Build history of the part. All positions in model axes, mm. A direction names the side the tool comes from. Give positions to 0.01 mm unless a question says otherwise; leave off trailing zeros. Write each loop counter-clockwise with the first axis right and the second up, starting at its lowest first coordinate (ties: lowest second). Pieces come first, ordered by that corner, then holes.
Autodesk Inventor part; units mm, degrees
ref_plane "YZ Plane" through (0, 0, 0) normal (1, 0, 0) x (0, 1, 0)
ref_plane "XZ Plane" through (0, 0, 0) normal (0, 1, 0) x (-1, 0, 0)
ref_plane "XY Plane" through (0, 0, 0) normal (0, 0, 1) x (1, 0, 0)
sketch "Sketch1" plane through (0, 0, 0) normal (0, 0, 1) x (1, 0, 0)
  line L0 (0, 0) -> (-40, 0)
  line L1 (-40, 0) -> (-40, -132)
  line L2 (-40, -132) -> (0, -132)
  line L3 (0, -132) -> (0, 0)
  line L4 (-30, -105) -> (-10, -105) construction
  line L5 (-10, -105) -> (-10, -125) construction
  line L6 (-10, -125) -> (-30, -125) construction
  line L7 (-30, -125) -> (-30, -105) construction
  line L8 (-20, -105) -> (-20, -80) construction
  line L9 (-20, -80) -> (-20, -60) construction
  line L10 (-20, -60) -> (-20, -40) construction
  line L11 (-20, -40) -> (-20, -20) construction
  line L12 (-20, -20) -> (-20, 0) construction
  dimension "d0" = 20
  dimension "d1" = 20
  dimension "d2" = 25
  dimension "d3" = 20
  dimension "d4" = 7
  dimension "d5" = 10
extrude "Plate1" add sketch "Sketch1" along normal blind 2.286
hole "Hole1" at (-20, -80, 0) at (-20, -60, 0) at (-20, -40, 0) at (-20, -20, 0) at (-10, -125, 0) at (-10, -105, 0) at (-30, -105, 0) at (-30, -125, 0) direction (0, 0, 1) diameter 3.4 end through all
sketch "Sketch2" plane through (-37.714, 0, 2.286) normal (-1, 0, 0) x (0, -1, 0)
  line L0 (132, 0) -> (0, 0)
  line L1 (0, 0) -> (0, -12.7)
  line L2 (0, -12.7) -> (132, -12.7)
  line L3 (132, -12.7) -> (132, 0)
edge flange "Flange1" height 12.7 angle 90 thickness 2.286 bend radius 2.286 thickness toward (-1, 0, 0) relief tear relief width 2.286 relief depth 1.143 corner gap 2.286 corner form 0 edges at (-40, -66, 0) (0, -66, 0) wall of the first edge with corners at (-37.714, -132, 2.286) (-37.714, 0, 2.286) (-37.714, 0, -10.414) (-37.714, -132, -10.414)
bend "Bend1"
corner "Corner1"
equation "\"d12\" = Thickness"
equation "\"d6\" = Thickness"
equation "\"d14\" = BendReliefWidth"
equation "\"d15\" = BendReliefDepth"
equation "\"d16\" = MinimumRemnant"
equation "\"d17\" = TransitionRadius"
equation "\"d20\" = BendRadius"
equation "\"d21\" = CornerReliefSize"
equation "\"d22\" = GapSize"
equation "\"d23\" = JacobiRadiusSize"
equation "\"BendRadius\" = Thickness"
equation "\"BendReliefWidth\" = Thickness"
equation "\"BendReliefDepth\" = 0.5 * Thickness"
equation "\"CornerReliefSize\" = 4 * Thickness"
equation "\"MinimumRemnant\" = 2 * Thickness"
equation "\"TransitionRadius\" = BendRadius"
equation "\"JacobiRadiusSize\" = BendRadius"
equation "\"GapSize\" = Thickness"
properties part number "Bed Mount"
(1) Drop flat-ended pins along their axis: pin 1 (4 mm diameter, centred on x = -22, y = -32, fed in from -Z); pin 2 (3 mm diameter, centred on x = -35.5, y = -40.5, fed in from -Z); pin 3 (6 mm diameter, centred on x = -33, z = -7.5, fed in from +Y). Give the stop position or say it passes through.
(2) Saw through at B-B, the plane z = -4. List the corners of the cut face in (x, y), plus the area to 3 significant figures.
(3) Saw through at C-C, the plane y = -20. List the corners of the cut face in (x, z), plus the area to 3 significant figures.
(4) Saw through at A-A, the plane x = -10. List the corners of the cut face in (y, z), plus the area to 3 significant figures.
(5) Probe line 1 (Y direction, x = -30, z = 0.55); line 2 (X direction, y = -23, z = -9.5); line 3 (X direction, y = -105, z = 1.1). List the from-to ranges inside material, lowest first.
(6) Saw through at D-D, the plane y = -105. List the corners of the cut face in (x, z).
(7) 3-axis set-ups, long thin cutter, end or side, ignore diameter. For faces 5 (the face through (-20, -65, 0)), 6 (the face through (-22, 0, 1)): which of +Z, -Z, +X, -X, +Y, -Y reach the whole face in a straight line?
(8) Mould opens along X. For faces 1 (the face through (-39, -65, -10.414)), 2 (the face through (-30.07, -106.7, 1.16)), 3 (the face through (-38.7, -65.08, 0.91)), 4 (the face through (0, -67, -6)) say: +X half, -X half, draft (parallel to the pull), parting line (faces both ways), or undercut.
Computed values:
1. pin 1: stops at z = 0
1. pin 2: stops at z = -0.63
1. pin 3: passes through
2. outline: (-40, -132) - (-37.71, -132) - (-37.71, 0) - (-40, 0) - close; (-2.29, -132) - (0, -132) - (0, 0) - (-2.29, 0) - close
2. area: 604 mm2
3. outline: (-40, -10.41) - (-37.71, -10.41) - (-37.71, -2.29) arc R2.29 cw to (-35.43, 0) - (-21.7, 0) - (-21.7, 2.29) - (-35.43, 2.29) arc R4.57 ccw to (-40, -2.29) - close; (-18.3, 0) - (-4.57, 0) arc R2.29 cw to (-2.29, -2.29) - (-2.29, -10.41) - (0, -10.41) - (0, -2.29) arc R4.57 ccw to (-4.57, 2.29) - (-18.3, 2.29) - close
3. area: 125 mm2
4. outline: (-132, 0) - (-126.7, 0) - (-126.7, 2.29) - (-132, 2.29) - close; (-123.3, 0) - (-106.7, 0) - (-106.7, 2.29) - (-123.3, 2.29) - close; (-103.3, 0) - (0, 0) - (0, 2.29) - (-103.3, 2.29) - close
4. area: 286 mm2
5. line 1: y = -132 to -126.7, -123.3 to -106.7, -103.3 to 0
5. line 2: x = -40 to -37.71, -2.29 to 0
5. line 3: x = -38.5 to -31.7, -28.3 to -11.7, -8.3 to -1.5
6. outline: (-40, -10.41) - (-37.71, -10.41) - (-37.71, -2.29) arc R2.29 cw to (-35.43, 0) - (-31.7, 0) - (-31.7, 2.29) - (-35.43, 2.29) arc R4.57 ccw to (-40, -2.29) - close; (-28.3, 0) - (-11.7, 0) - (-11.7, 2.29) - (-28.3, 2.29) - close; (-8.3, 0) - (-4.57, 0) arc R2.29 cw to (-2.29, -2.29) - (-2.29, -10.41) - (0, -10.41) - (0, -2.29) arc R4.57 ccw to (-4.57, 2.29) - (-8.3, 2.29) - close
7. face 5: -Z, +Y, -Y
7. face 6: +Z, -Z, +X, -X, +Y
8. face 1: draft
8. face 2: undercut
8. face 3: -X half
8. face 4: +X half
